from build123d import *

# Parameters (mm, degrees)
SKETCH1_W           = 304.8
SKETCH1_H           = 203.2
SKETCH1_R           = 14.2875
SKETCH1_R_2         = 9.525
SKETCH1_R_3         = 2.54
BOSS_EXTRUDE1_DEPTH = 12.7
SKETCH5_R           = 2.38379
CUT_EXTRUDE2_DEPTH  = 475.681082412


with BuildPart() as part:
    # Sketch1 → Boss-Extrude1 (new body)
    with BuildSketch(Plane(origin=(0, 0, 0), x_dir=(1, 0, 0), z_dir=(0, 1, 0))):
        with Locations((0, -25.4)):
            Rectangle(SKETCH1_W, SKETCH1_H)
        with Locations(Location((0, 0, 0), (0, 0, 270))):
            Circle(SKETCH1_R, mode=Mode.SUBTRACT)
        with Locations(Location((-53.34, 0, 0), (0, 0, 270))):
            Circle(SKETCH1_R_2, mode=Mode.SUBTRACT)
        with Locations(Location((-53.34, 25.4, 0), (0, 0, 270))):
            Circle(SKETCH1_R_3, mode=Mode.SUBTRACT)
        with Locations(Location((-53.34, -25.4, 0), (0, 0, 270))):
            Circle(SKETCH1_R_3, mode=Mode.SUBTRACT)
    boss_extrude1 = extrude(amount=BOSS_EXTRUDE1_DEPTH)

    # Mirror1: Boss-Extrude1 across plane
    add(boss_extrude1.mirror(Plane(origin=(152.4, 12.7, -76.2), x_dir=(0, 0, 1), z_dir=(-1, 0, 0))))

    # Sketch5 → Cut-Extrude2 (cut, through all)
    with BuildSketch(Plane(origin=(0, 12.7, 0), x_dir=(1, 0, 0), z_dir=(0, 1, 0))):
        with Locations(Location((157.48, 65.607045243, 0), (0, 0, 270))):
            Circle(SKETCH5_R)
        with Locations(Location((147.32, 65.607045243, 0), (0, 0, 270))):
            Circle(SKETCH5_R)
        with Locations(Location((147.32, 17.982045243, 0), (0, 0, 270))):
            Circle(SKETCH5_R)
        with Locations(Location((157.48, 17.982045243, 0), (0, 0, 270))):
            Circle(SKETCH5_R)
        with BuildLine():
            Line((142.4305, 21.792045243), (162.3695, 21.792045243))
            ThreePointArc((162.3695, 21.792045243), (164.7571, 24.179645243), (162.3695, 26.567245243))
            Line((162.3695, 26.567245243), (162.3695, 57.021845243))
            ThreePointArc((162.3695, 57.021845243), (164.7571, 59.409445243), (162.3695, 61.797045243))
            Line((162.3695, 61.797045243), (142.4305, 61.797045243))
            ThreePointArc((142.4305, 61.797045243), (140.0429, 59.409445243), (142.4305, 57.021845243))
            Line((142.4305, 57.021845243), (142.4305, 26.567245243))
            ThreePointArc((142.4305, 26.567245243), (140.0429, 24.179645243), (142.4305, 21.792045243))
        make_face()
    extrude(amount=-CUT_EXTRUDE2_DEPTH, mode=Mode.SUBTRACT)


solid = part.part
Part model, mm, in its own coordinate system. A direction names the side the tool comes from. Give positions to 0.01 mm unless a question says otherwise; leave off trailing zeros. Loops run counter-clockwise (first coordinate to the right, second up) from the corner with the lowest first, then second, coordinate; pieces in that order, holes last. Notation, with made-up numbers: M 78.25,62 L 87.25,62 A38 ccw 87.25,101 Z; hole C 31.25,41.25 d6. An arc over 180 degrees is marked long. Put each result on its own line as item: value. Start each with the question number.
1) Saw through at A-A (z = 0). List the corners of the cut face in (x, y) (1 decimal).
2) Probe probe 1 along X at (y, z) = (5, 25.4); probe 2 along Z at (x, y) = (147.32, 3); probe 3 along X at (y, z) = (7.25, 0) (1 decimal). List the from-to ranges inside material, lowest first.
3) 3-axis set-ups, long thin cutter, end or side, ignore diameter. For faces 4 (the flat face through (142.43, 6, -42)), 5 (the flat face through (157, 12.7, 24)): which of +Z, -Z, +X, -X, +Y, -Y reach the whole face in a straight line?
4) Pull direction Z, two halves, no side cores. Call faces 1 (the flat face through (157, 6, 127)), 2 (the flat face through (-152.4, 6, 27)), 3 (the flat face through (162.37, 6, -42)): +Z half, -Z half, draft (parallel to the pull), parting line (faces both ways), or undercut.
5) Flat gauge pin, fed straight in: pin 1 (4.5 mm diameter, centred on x = -53.34, z = -25.4, fed in from +Y). Where does the tip first touch, or does it go through?
6) Saw through at B-B (y = 5.75). State how many separate pieces and enclosed holes the cut face has, then the cut area to 3 significant figures.
Numbers:
1. outline: M -152.4,0 L -62.9,0 L -62.9,12.7 L -152.4,12.7 Z; M -43.8,0 L -14.3,0 L -14.3,12.7 L -43.8,12.7 Z; M 14.3,0 L 290.5,0 L 290.5,12.7 L 14.3,12.7 Z; M 319.1,0 L 348.6,0 L 348.6,12.7 L 319.1,12.7 Z; M 367.7,0 L 457.2,0 L 457.2,12.7 L 367.7,12.7 Z
2. probe 1: -152.4 to -55.88, -50.8 to 355.6, 360.68 to 457.2
2. probe 2: -76.2 to -67.99, -63.22 to -61.8, -21.79 to -20.37, -15.6 to 127
2. probe 3: -152.4 to -62.9, -43.8 to -14.3, 14.3 to 290.5, 319.1 to 348.6, 367.7 to 457.2
3. face 4: +Y, -Y
3. face 5: +Z, -Z, +X, -X, +Y
4. face 1: +Z half
4. face 2: draft
4. face 3: undercut
5. pin 1: through
6. separate pieces: 1
6. enclosed holes: 13
6. area: 121,000 mm^2
